```python
from build123d import *

# Parameters (mm, degrees)
F0_R     = 6.3754
F1_DEPTH = 9.525
F2_R     = 2.54
F3_R     = 2.54


with BuildPart() as f1:
    # F0 (on Front) → F1 (new body)
    with BuildSketch(Plane.XZ):
        with BuildLine():
            ThreePointArc((20.258996, 9.87189), (22.492237, 21.066453), (33.413953, 24.386349))
            Line((33.413953, 24.386349), (20.62332, 37.176983))
            Line((20.62332, 37.176983), (-8.562513, 7.99115))
            ThreePointArc((-8.562513, 7.99115), (-12.282257, -0.989106), (-8.562513, -9.969362))
            Line((-8.562513, -9.969362), (18.922999, -37.454874))
            Line((18.922999, -37.454874), (78.158512, -37.454874))
            Line((78.158512, -37.454874), (78.158512, -31.104874))
            Line((78.158512, -31.104874), (84.508512, -31.104874))
            Line((84.508512, -31.104874), (84.508512, -37.454874))
            Line((84.508512, -37.454874), (103.558512, -37.454874))
            Line((103.558512, -37.454874), (103.558512, -31.104874))
            Line((103.558512, -31.104874), (109.908512, -31.104874))
            Line((109.908512, -31.104874), (109.908512, -37.454874))
            Line((109.908512, -37.454874), (116.258512, -37.454874))
            Line((116.258512, -37.454874), (116.258512, -18.404874))
            Line((116.258512, -18.404874), (35.794024, -18.404874))
            Line((35.794024, -18.404874), (13.888128, 3.501022))
            Line((13.888128, 3.501022), (20.258996, 9.87189))
        make_face()
        with Locations((0.417743, -0.989106)):
            Circle(F0_R, mode=Mode.SUBTRACT)
    extrude(amount=-F1_DEPTH)

    # F2
    f2_edges = [f1.edges().sort_by_distance(p)[0] for p in [
        (33.413953, 4.7625, 24.386349),
        (20.258996, 4.7625, 9.87189),
    ]]
    fillet(f2_edges, radius=F2_R)

    # F3
    f3_edges = [f1.edges().sort_by_distance(p)[0] for p in [
        (13.888128, 4.7625, 3.501022),
        (35.794024, 4.7625, -18.404874),
        (18.922999, 4.7625, -37.454874),
        (116.258512, 4.7625, -18.404874),
        (116.258512, 4.7625, -37.454874),
        (20.62332, 4.7625, 37.176983),
    ]]
    fillet(f3_edges, radius=F3_R)


solid = f1.part
```
The model under review builds one solid part; all positions refer to its coordinate system, in mm. A direction names the side the tool comes from. Coordinates: 2 decimals unless noted, no trailing zeros. Write each loop counter-clockwise with the first axis right and the second up, starting at its lowest first coordinate (ties: lowest second). Pieces come first, ordered by that corner, then holes. Notation, with made-up numbers: (20, 87) -> (64, 87) arc R14 ccw to (64, 97) -> close; hole circle Ø11 at (63.5, -19.5). An arc over 180 degrees is marked (long way). One line per item, written item: value. Start each with the question number.
Q1. To check wall thickness, follow probe 1 along Z at (x, y) = (91, 5.25); probe 2 along Z at (x, y) = (84, 8); probe 3 along Z at (x, y) = (25, 4.5). State the ranges of each line that lie inside material, in increasing order.
Q2. The part is to be moulded in two halves that separate along Z. For faces 4 (the face through (29.8, 4.8, 26.1)), 5 (the face through (25.8, 4.7, 32)), 6 (the face through (49, 5, -37.455)), say which applies: +Z half, -Z half, draft (parallel to the pull), parting line (faces both ways), or undercut.
Q3. For faces 1 (the face through (42, 0, -20)), 2 (the face through (17.418, 4.696, 7.031)), 3 (the face through (103.559, 5, -34)), list the 3-axis set-ups (+Z, -Z, +X, -X, +Y, -Y) from which the entire face can be reached by the end or side of a thin tool; tool diameter is ignored.
Q4. Add section A-A, the plane x = 4. Give the boundary of the cut face in (y, z) (3 decimals), then the cut area to 3 significant figures.
Q5. Add section B-B, the plane z = -3.5. Give the boundary of the cut face in (x, y) (3 decimals), then the cut area to 3 significant figures.
Q6. Add section C-C, the plane y = 2.25. Give the boundary of the cut face in (x, z) (1 decimal), then the cut area to 3 significant figures.
Q7. Clearance check with flat-ended pins moving along their axes: P1, Ø2, axis at y = 3, z = 3, coming from the -X side; P2, Ø3, axis at y = 5, z = -7.5, coming from the -X side; P3, Ø5, axis at y = 3.5, z = -35.5, coming from the -X side; P4, Ø14.5, axis at x = 0.42, z = -0.99, coming from the -Y side. State where each tip first meets the part, or that it passes through.
Q8. Add section D-D, the plane x = 80.5. Give the boundary of the cut face in (y, z) (3 decimals), then the cut area to 3 significant figures.
Response:
1. probe 1: -37.45 to -18.4
1. probe 2: -31.1 to -18.4
1. probe 3: -37.45 to -7.61, 23.13 to 32.8
2. face 4: undercut
2. face 5: +Z half
2. face 6: -Z half
3. face 1: +Z, -Z, +X, -X, -Y
3. face 2: +X, +Y, -Y
3. face 3: -Z, +Y, -Y
4. outline: (0, -22.532) -> (9.525, -22.532) -> (9.525, -6.263) -> (0, -6.263) -> close; (0, 4.285) -> (9.525, 4.285) -> (9.525, 20.554) -> (0, 20.554) -> close
4. area: 310 mm²
5. outline: (-12.032, 0) -> (-5.442, 0) -> (-5.442, 9.525) -> (-12.032, 9.525) -> close; (6.278, 0) -> (20.889, 0) -> (20.889, 9.525) -> (6.278, 9.525) -> close
5. area: 202 mm²
6. outline: (-8.6, -10) -> (18.2, -36.7) arc R2.5 ccw to (20, -37.5) -> (78.2, -37.5) -> (78.2, -31.1) -> (84.5, -31.1) -> (84.5, -37.5) -> (103.6, -37.5) -> (103.6, -31.1) -> (109.9, -31.1) -> (109.9, -37.5) -> (113.7, -37.5) arc R2.5 ccw to (116.3, -34.9) -> (116.3, -20.9) arc R2.5 ccw to (113.7, -18.4) -> (36.8, -18.4) arc R2.5 cw to (35.1, -17.7) -> (15.7, 1.7) arc R2.5 cw to (15.7, 5.3) -> (19.2, 8.8) arc R2.5 ccw to (19.9, 11.2) arc R11.1 cw to (28, 24.4) arc R2.5 ccw to (29.2, 28.6) -> (22.4, 35.4) arc R2.5 ccw to (18.8, 35.4) -> (-8.6, 8) arc R12.7 ccw to start; hole circle Ø12.8 at (0.4, -1)
6. area: 3,180 mm²
7. P1: x = -11.93
7. P2: x = -11.25
7. P3: x = 14.47
7. P4: y = 0
8. outline: (0, -31.105) -> (9.525, -31.105) -> (9.525, -18.405) -> (0, -18.405) -> close
8. area: 121 mm²
